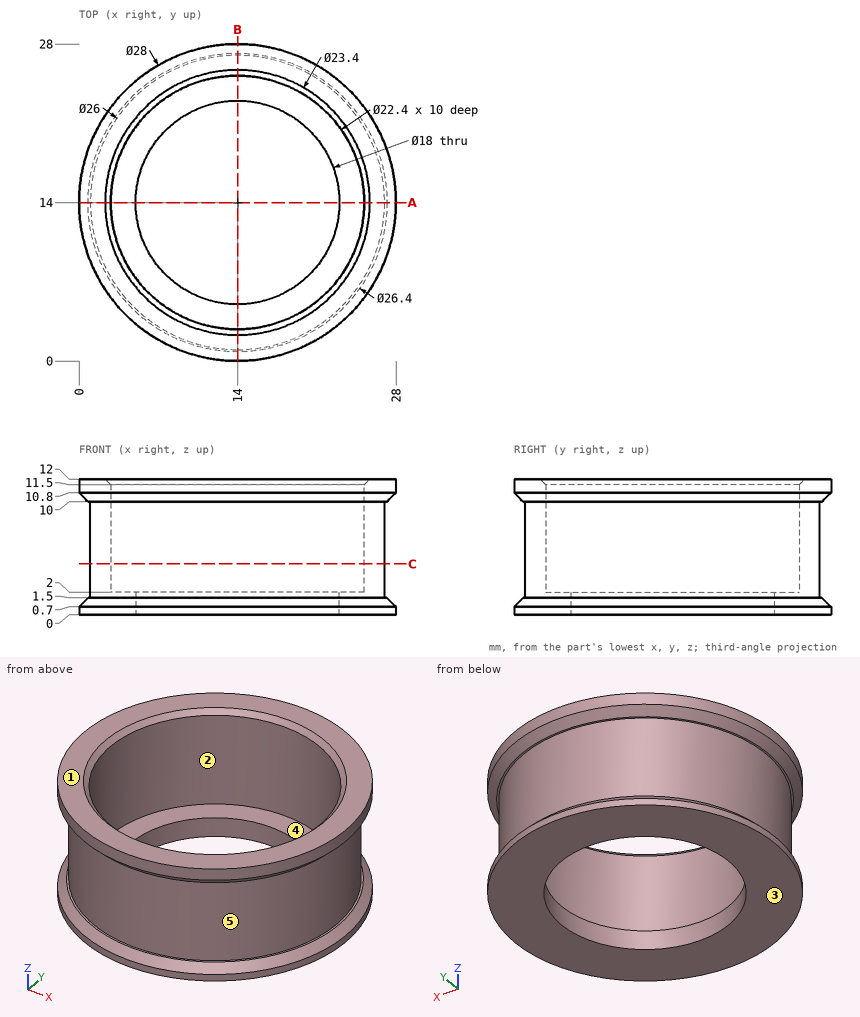
Geometry: see drawing. Coordinates: mm, zero at the bounding-box minimum. A direction names the side the tool comes from. Give positions to 0.01 mm unless a question says otherwise; leave off trailing zeros. Loops run counter-clockwise (first coordinate to the right, second up) from the corner with the lowest first, then second, coordinate; pieces in that order, holes last. Notation, with made-up numbers: (11, 13.5) - (49, 13.5) arc R14 cw to (49, 37.5) - close; hole circle Ø4 at (51.25, 25). An arc over 180 degrees is marked (long way). Use CSV: the item, a comma, the result in double quotes.
1) Cut plane A-A (y = 14). Output: boundary loops of the cut face in (x, z).
Worked out:
outline,"(0, 0) - (5, 0) - (5, 2) - (2.8, 2) - (2.8, 11.5) - (2.3, 12) - (0, 12) - (0, 10.8) - (0.8, 10) - (1, 10) - (1, 1.5) - (0.8, 1.5) - (0, 0.7) - close; (23, 0) - (28, 0) - (28, 0.7) - (27.2, 1.5) - (27, 1.5) - (27, 10) - (27.2, 10) - (28, 10.8) - (28, 12) - (25.7, 12) - (25.2, 11.5) - (25.2, 2) - (23, 2) - close"
2) Line query: line 1 (X direction, y = 14, z = 4.5); line 2 (Y direction, x = 14, z = 0.6); line 3 (Y direction, x = 14, z = 0.8). Output: solid intervals per line, ascending.
Worked out:
line 1,"x = 1 to 2.8, 25.2 to 27"
line 2,"y = 0 to 5, 23 to 28"
line 3,"y = 0.1 to 5, 23 to 27.9"
3) Pin query (flat end, axial travel): P1, Ø6, axis at y = 10, z = 7, coming from the -X side; P2, Ø3, axis at y = 15.5, z = 10, coming from the -X side; P3, Ø11, axis at x = 18.5, y = 16.5, coming from the +Z side. Return the tip coordinate at first contact, or that it passes through.
Worked out:
P1,"stops at x = 1.04"
P2,"stops at x = 0"
P3,"stops at z = 2"
4) Cut plane C-C (z = 4.5). Output: boundary loops of the cut face in (x, y), and give its area (3 significant figures).
Worked out:
outline,"circle Ø26 at (14, 14); hole circle Ø22.4 at (14, 14)"
area,"137 mm^2"
5) Mould query, pull axis Y, two halves, no side actions, for the marked faces 3, 4 and 5. Classes: +Y half, -Y half, draft (parallel to the pull), parting line (faces both ways), or undercut.
Worked out:
face 3,"draft"
face 4,"undercut"
face 5,"parting line"
6) Set-up query: the marked faces 1 and 2. Return all of +Z, -Z, +X, -X, +Y, -Y with unobstructed straight access to the full face (end or side cutting, diameter ignored); none if empty.
Worked out:
face 1,"+Z, +X, -X, +Y, -Y"
face 2,"+Z"
